from build123d import *

# Parameters (mm, degrees)
BOSS_EXTRUDE1_START = -0.046461
SKETCH4_R           = 0.666231497
BOSS_EXTRUDE1_DEPTH = 0.846461
CHAMFER1_SIZE       = 0.3
FILLET1_R           = 0.2
CHAMFER2_SIZE       = 0.4
SKETCH5_R           = 0.55
BOSS_EXTRUDE2_DEPTH = 4.9
SKETCH5_3_R         = 0.8
BOSS_EXTRUDE3_DEPTH = 4.5


with BuildPart() as part:
    # Sketch1 → Revolve1 (revolve)
    with BuildSketch(Plane(origin=(0, 0, 0), x_dir=(0, 0, -1), z_dir=(1, 0, 0))):
        Polygon((0, 0), (0, 2), (0.286334312, 2), (0.286334312, 9.384488656), (1.723916807, 9.384488656), (1.723916807, 2), (4.3, 2), (4.3, 13.7), (4.8, 13.7), (4.8, 2), (5.5, 2), (5.5, 0), align=None)
    revolve(axis=Axis((0, 0, 0), (0, 1, 0)))

    # Sketch4 → Boss-Extrude1 (add)
    with BuildSketch(Plane.XY.offset(4.8).offset(BOSS_EXTRUDE1_START)):
        with Locations((0, 10.320424239)):
            Circle(SKETCH4_R)
    boss_extrude1 = extrude(amount=BOSS_EXTRUDE1_DEPTH)

    # Mirror1: Boss-Extrude1 across plane
    add(boss_extrude1.mirror(Plane(origin=(0, 0, 0), x_dir=(1, 0, 0), z_dir=(0, 0, -1))))

    # Chamfer1
    chamfer1_edges = [part.edges().sort_by_distance(p)[0] for p in [
        (0, 2, 5.5),
    ]]
    chamfer(chamfer1_edges, length=CHAMFER1_SIZE)

    # Fillet1
    fillet1_edges = [part.edges().sort_by_distance(p)[0] for p in [
        (0, 9.384488656, 0.286334312),
    ]]
    fillet(fillet1_edges, radius=FILLET1_R)

    # Chamfer2
    chamfer2_edges = [part.edges().sort_by_distance(p)[0] for p in [
        (0, 9.384488656, 1.723916807),
    ]]
    chamfer(chamfer2_edges, length=CHAMFER2_SIZE)

    # Sketch5 → Boss-Extrude2 (add)
    with BuildSketch(Plane.XZ):
        with Locations(Location((0, 0, 0), (0, 0, 270))):
            Circle(SKETCH5_R)
    extrude(amount=BOSS_EXTRUDE2_DEPTH)

    # Sketch5<3> → Boss-Extrude3 (add)
    with BuildSketch(Plane.XZ):
        with Locations(Location((-3.13, 3.13, 0), (0, 0, 270))):
            Circle(SKETCH5_3_R)
        with Locations(Location((3.13, 3.13, 0), (0, 0, 270))):
            Circle(SKETCH5_3_R)
        with Locations(Location((-3.13, -3.13, 0), (0, 0, 270))):
            Circle(SKETCH5_3_R)
        with Locations(Location((3.13, -3.13, 0), (0, 0, 270))):
            Circle(SKETCH5_3_R)
    extrude(amount=BOSS_EXTRUDE3_DEPTH)


solid = part.part
Design review of the part built by this model. Coordinates are the model's own, in mm. A direction names the side the tool comes from. Coordinates: 2 decimals unless noted, no trailing zeros. Order: outer loops, then holes, each group sorted by start corner. A loop starts at its lowest first (then second) coordinate and runs counter-clockwise, first axis right, second up. Notation, with made-up numbers: (82, -30.5) -> (120, -30.5) arc R20 ccw to (120, -23.5) -> close; hole circle Ø9 at (42, 3). An arc over 180 degrees is marked (long way). One line per item, written item: value.
1) We need section B-B, the plane y = 7.75. Give the boundary of the cut face in (x, z).
Output values:
outline: circle Ø9.6 at (0, 0); circle Ø3.45 at (0, 0); hole circle Ø8.6 at (0, 0); hole circle Ø0.57 at (0, 0)
2) Machinability: for faces 1 (the face through (3.37, -2.218, 2.367)), 2 (the face through (0, 9.384, 1)), 3 (the face through (-3, -4.5, -3)), 4 (the face through (0.615, 10.065, 5.171)), which of the approach directions +Z, -Z, +X, -X, +Y, -Y give a long, thin tool a straight path to every point of the face, cutting with its end or side? Answer none if there is none.
Output values:
face 1: -Y
face 2: +Y
face 3: +Z, -Z, +X, -X, -Y
face 4: +Z
3) To check wall thickness, follow probe 1 along X at (y, z) = (4.25, 0); probe 2 along Z at (x, y) = (0.75, 3). State the ranges of each line that lie inside material, in increasing order. Write a range as [from, to].
Output values:
probe 1: x = [-4.8, -4.3], [-1.72, -0.29], [0.29, 1.72], [4.3, 4.8]
probe 2: z = [-4.74, -4.23], [-1.55, 1.55], [4.23, 4.74]
4) We need section A-A, the plane y = -0.5. Give the boundary of the cut face in (x, z).
Output values:
outline: circle Ø1.6 at (-3.13, -3.13); circle Ø1.6 at (-3.13, 3.13); circle Ø1.1 at (0, 0); circle Ø1.6 at (3.13, -3.13); circle Ø1.6 at (3.13, 3.13)
5) Clearance check with flat-ended pins moving along their axes: P1, Ø0.8, axis at x = 3.5, z = -3, coming from the -Y side; P2, Ø4, axis at x = 4, z = 0, coming from the +Y side; P3, Ø3, axis at x = 0, z = 0, coming from the +Y side; P4, Ø1.5, axis at y = 3.5, z = 0, coming from the +X side. State where each tip first meets the part, or that it passes through.
Output values:
P1: stops at y = -4.5
P2: stops at y = 13.7
P3: stops at y = 9.38
P4: stops at x = 4.8
6) Draft analysis for pull direction Y (two halves, no side actions). For faces 5 (the face through (2, 2, 0)), 6 (the face through (0.615, 10.065, -5.171)), 7 (the face through (0, 10, -5.6)), 8 (the face through (0, 0, -1)), state which applies: +Y half, -Y half, draft (parallel to the pull), parting line (faces both ways), or undercut.
Output values:
face 5: +Y half
face 6: undercut
face 7: draft
face 8: -Y half
